Model file for the job. Use its own axes, mm. A direction names the side the tool comes from. Give positions to 0.01 mm unless a question says otherwise; leave off trailing zeros. Write each loop counter-clockwise with the first axis right and the second up, starting at its lowest first coordinate (ties: lowest second). Pieces come first, ordered by that corner, then holes.
Autodesk Inventor part; units mm, degrees
ref_plane "YZ Plane" through (0, 0, 0) normal (1, 0, 0) x (0, 1, 0)
ref_plane "XZ Plane" through (0, 0, 0) normal (0, 1, 0) x (-1, 0, 0)
ref_plane "XY Plane" through (0, 0, 0) normal (0, 0, 1) x (1, 0, 0)
sketch "Sketch1" plane through (0, 0, 0) normal (0, 1, 0) x (-1, 0, 0)
  circle A0 centre (0, 0) radius 11.5
  dimension "d0" = 23
extrude "Extrusion1" add sketch "Sketch1" along normal blind 15
sketch "Sketch2" plane through (0, 0, 0) normal (1, 0, 0) x (0, 1, 0)
  line L0 (0, 0) -> (20.5, 0)
  line L1 (20.5, 0) -> (11.0014, 0) construction
  line L2 (20.5, 0) -> (29.9986, 0) construction
  arc A0 (20.5, 0) -> (15, 8.616) centre (11.0014, 0) ccw
  line L3 (15, 8.616) -> (15, 0)
  line L4 (15, -11.5) -> (15, 11.5)
  line L5 (15, 8.616) -> (15, 0)
  line L6 (20.5, 0) -> (15, 0)
  arc A1 (20.5, 0) -> (15, 8.616) centre (11.0014, 0) ccw
  dimension "d3" = 20.5
  dimension "d4" = 9.4986
  dimension "d5" = 180
revolve "Revolution1" add sketch "Sketch2" angle 360 about axis through (0, 20.5, 0) along (0, 1, 0)
sketch "Sketch3" plane through (0, 0, 0) normal (0, -1, 0) x (1, 0, 0)
  line L0 (0, 0) -> (0, -7.5) construction
  line L1 (0, -7.5) -> (0, 7.5)
  circle A0 centre (0, 7.5) radius 1.25
  circle A1 centre (0, -7.5) radius 1.25
  dimension "d7" = 7.5
  dimension "d8" = 15
  dimension "d9" = 2.5
  dimension "d10" = 2.5
extrude "Extrusion2" cut sketch "Sketch3" against normal blind 5
properties part number "Caster"
1. Pin check, flat tips, straight feed: P1, Ø12, axis at y = 14, z = -4, coming from the +X side; P2, Ø0.8, axis at x = 0, z = 8, coming from the -Y side; P3, Ø2, axis at y = 8, z = 7.5, coming from the +X side; P4, Ø8, axis at x = 7, y = 9.5, coming from the +Z side. Stop position of each tip, or through.
Calculated:
P1: stops at x = 11.5
P2: stops at y = 5
P3: stops at x = 9.49
P4: stops at z = 11.1
2. Slice it at B-B, the plane y = 12. Write the cut outline in (x, z).
Calculated:
outline: circle Ø23 at (0, 0)
3. Pull direction X, two halves, no side cores. Call faces 3 (the flat face through (0, 0, 0)), 4 (the cylindrical face through (1.5, 7.4, -11.4)), 5 (the flat face through (0, 5, 8)): +X half, -X half, draft (parallel to the pull), parting line (faces both ways), or undercut.
Calculated:
face 3: draft
face 4: parting line
face 5: undercut
4. Which spindle directions (+Z, -Z, +X, -X, +Y, -Y) get a long thin tool onto all of the face, cutting with end or side? Do faces 1 (the flat face through (0, 5, -7)), 2 (the flat face through (1, 15, 9)). Say none if no direction does.
Calculated:
face 1: -Y
face 2: +Y
5. Slice it at A-A, the plane y = 2.25. Write the cut outline in (x, z).
Calculated:
outline: circle Ø23 at (0, 0); hole circle Ø2.5 at (0, -7.5); hole circle Ø2.5 at (0, 7.5)
6. Probe probe 1 along Z at (x, y) = (0, 3.2); probe 2 along Y at (x, z) = (2.75, -10.5); probe 3 along X at (y, z) = (2.1, -7.5). List the from-to ranges inside material, lowest first.
Calculated:
probe 1: z = -11.5 to -8.75, -6.25 to 6.25, 8.75 to 11.5
probe 2: y = 0 to 15
probe 3: x = -8.72 to -1.25, 1.25 to 8.72
